Can you work these out from the model? Positions are in its coordinate system, mm. Coordinates: 2 decimals unless noted, no trailing zeros.
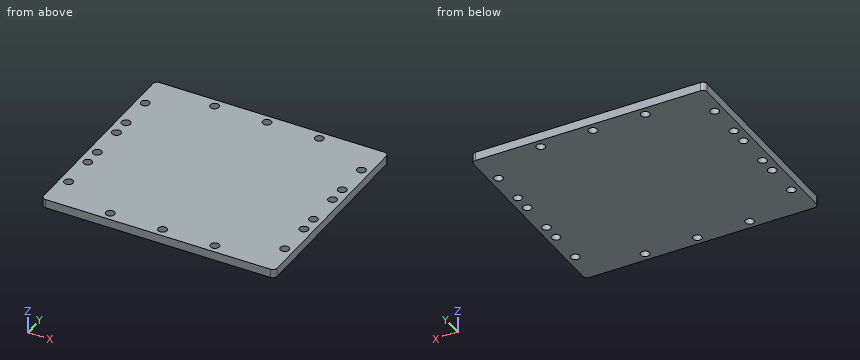
```python
from build123d import *

# Parameters (mm, degrees)
SKETCH_1_R      = 1
EXTRUDE_1_DEPTH = 2


with BuildPart() as part:
    # 草圖1 → 填料-伸長1 (new body)
    with BuildSketch(Plane.XY):
        with BuildLine():
            Line((-35.200489897, 20.825), (16.399510103, 20.825))
            ThreePointArc((16.399510103, 20.825), (17.106616884, 20.532106781), (17.399510103, 19.825))
            Line((17.399510103, 19.825), (17.399510103, -25.775))
            ThreePointArc((17.399510103, -25.775), (17.106616884, -26.482106781), (16.399510103, -26.775))
            Line((16.399510103, -26.775), (-35.200489897, -26.775))
            ThreePointArc((-35.200489897, -26.775), (-35.907596678, -26.482106781), (-36.200489897, -25.775))
            Line((-36.200489897, -25.775), (-36.200489897, 19.825))
            ThreePointArc((-36.200489897, 19.825), (-35.907596678, 20.532106781), (-35.200489897, 20.825))
        make_face()
        with Locations((-9.450489897, 18.825)):
            Circle(SKETCH_1_R, mode=Mode.SUBTRACT)
        with Locations((-9.450489897, -24.775)):
            Circle(SKETCH_1_R, mode=Mode.SUBTRACT)
        with Locations((15.399510103, 1.025)):
            Circle(SKETCH_1_R, mode=Mode.SUBTRACT)
        with Locations((-34.200489897, 1.025)):
            Circle(SKETCH_1_R, mode=Mode.SUBTRACT)
        with Locations((-34.200489897, -6.975)):
            Circle(SKETCH_1_R, mode=Mode.SUBTRACT)
        with Locations((15.399510103, -6.975)):
            Circle(SKETCH_1_R, mode=Mode.SUBTRACT)
        with Locations((-34.200489897, 13.025)):
            Circle(SKETCH_1_R, mode=Mode.SUBTRACT)
        with Locations((-34.200489897, 5.025)):
            Circle(SKETCH_1_R, mode=Mode.SUBTRACT)
        with Locations((-34.200489897, -10.975)):
            Circle(SKETCH_1_R, mode=Mode.SUBTRACT)
        with Locations((-34.200489897, -18.975)):
            Circle(SKETCH_1_R, mode=Mode.SUBTRACT)
        with Locations((15.399510103, 13.025)):
            Circle(SKETCH_1_R, mode=Mode.SUBTRACT)
        with Locations((15.399510103, 5.025)):
            Circle(SKETCH_1_R, mode=Mode.SUBTRACT)
        with Locations((15.399510103, -10.975)):
            Circle(SKETCH_1_R, mode=Mode.SUBTRACT)
        with Locations((15.399510103, -18.975)):
            Circle(SKETCH_1_R, mode=Mode.SUBTRACT)
        with Locations((-21.450489897, 18.825)):
            Circle(SKETCH_1_R, mode=Mode.SUBTRACT)
        with Locations((2.549510103, 18.825)):
            Circle(SKETCH_1_R, mode=Mode.SUBTRACT)
        with Locations((-21.450489897, -24.775)):
            Circle(SKETCH_1_R, mode=Mode.SUBTRACT)
        with Locations((2.549510103, -24.775)):
            Circle(SKETCH_1_R, mode=Mode.SUBTRACT)
    extrude(amount=EXTRUDE_1_DEPTH)


solid = part.part
```
Item 1: I'm going to push a flat-ended pin straight in: P1, Ø1.8, axis at x = -34.2, y = -10.98, coming from the +Z side. Where does the tip first touch, or does it pass through?
Results are:
P1: passes through
Item 2: I need wall thicknesses on line 1 along X through (y, z) = (-24, 0.3); line 2 along X through (y, z) = (-7.5, 0.45); line 3 along Y through (x, z) = (-9, 1.5) (3 decimals). Which ranges of each line are inside material? Lowest first, please.
Results are:
line 1: x = -36.2 to -22.08, -20.82 to -10.08, -8.82 to 1.92, 3.18 to 17.4
line 2: x = -36.2 to -35.05, -33.35 to 14.55, 16.25 to 17.4
line 3: y = -26.775 to -25.668, -23.882 to 17.932, 19.718 to 20.825
Item 3: Suppose I cut it at A-A, the plane z = 1.3. Count the separate pieces of the cut face and the enclosed holes in it, plus the area to 3 significant figures.
Results are:
separate pieces: 1
enclosed holes: 18
area: 2,490 mm2
